CAD build for the part. Positions are in the model's coordinates, mm. Face numbers are marked on the shaded views. A direction names the side the tool comes from. Give positions to 0.01 mm unless a question says otherwise; leave off trailing zeros. Loops run counter-clockwise (first coordinate to the right, second up) from the corner with the lowest first, then second, coordinate; pieces in that order, holes last. Notation, with made-up numbers: (67.25, -10.5) -> (87.25, -10.5) arc R28 ccw to (87.25, 16.5) -> close; hole circle Ø2 at (-21, -11.5). An arc over 180 degrees is marked (long way). Write each question's results on one line, items separated by ' | '. Start each with the question number.
```python
from build123d import *

# Parameters (mm, degrees)
F0_R     = 8.5
F0_R_2   = 5
F1_DEPTH = 6
F2_DEPTH = 11.5
F4_D     = 3.3
F4_DEPTH = 10.001
F5_D     = 3.3


with BuildPart() as f1:
    # F0 (on Front) → F1 (new body)
    with BuildSketch(Plane.XZ):
        with BuildLine():
            Line((-1.5, 11.9058808998), (-5, 8.6602540378))
            ThreePointArc((-5, 8.6602540378), (0, -10), (5, 8.6602540378))
            Line((5, 8.6602540378), (1.5, 11.9058808998))
            ThreePointArc((1.5, 11.9058808998), (0, 12), (-1.5, 11.9058808998))
        make_face()
        Circle(F0_R, mode=Mode.SUBTRACT)
        Circle(F0_R)
        Circle(F0_R_2, mode=Mode.SUBTRACT)
    extrude(amount=F1_DEPTH)

    # F0 (on Front) → F2 (join)
    with BuildSketch(Plane.XZ):
        Circle(F0_R)
        Circle(F0_R_2, mode=Mode.SUBTRACT)
    extrude(amount=F2_DEPTH)

    # F4 (through all, one way)
    with BuildSketch(Plane.YZ):
        with Locations((-8.75, 0)):
            Circle(F4_D / 2)
    extrude(amount=-F4_DEPTH, mode=Mode.SUBTRACT)

    # F5 (through all)
    with Locations(Plane(origin=(0, 0, 0), x_dir=(0, 1, 0), z_dir=(-1, 0, 0))):
        with Locations((-8.75, 0)):
            Hole(F5_D / 2)


solid = f1.part
```
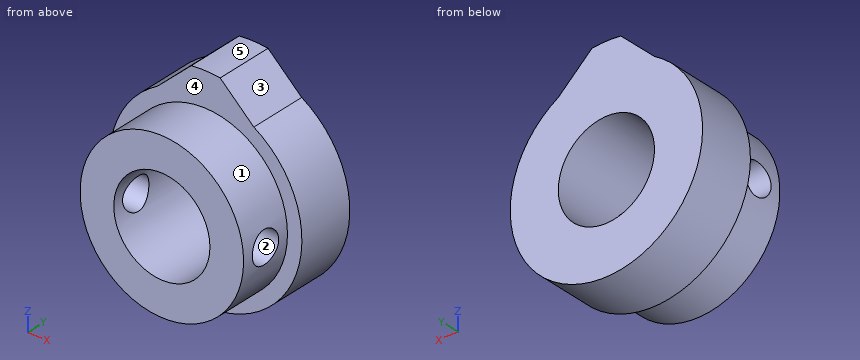
Q1. Mould opens along Z. For the marked faces 1, 2 and 3 say: pulls with the +Z half, pulls with the -Z half, needs draft (parallel to the pull), parting line crosses it, or undercut.
Q2. Saw through at B-B, the plane z = 0.5. List the corners of the cut face in (x, y).
Q3. Saw through at A-A, the plane x = 0. List the corners of the cut face in (y, z), then the cut area to 4 significant figures.
Q4. Saw through at C-C, the plane y = -8.75. List the corners of the cut face in (x, z), then the cut area to 3 significant figures.
Q5. Saw through at D-D, the plane z = -3.75. List the corners of the cut face in (x, y).
Q6. Wall check: L1, parallel to Z at x = 0, y = -3.5; L2, parallel to Z at x = 3.5, y = -6.25; L3, parallel to X at y = -2.25, z = 0. Give the ranges that are in metal, low to high.
Q7. Drop flat-ended pins along their axis: pin 1 (4 mm diameter, centred on x = -5.5, y = -8.5, fed in from -Z); pin 2 (8 mm diameter, centred on x = -3.5, z = 4, fed in from +Y); pin 3 (2 mm diameter, centred on y = -10, z = 4.5, fed in from -X); pin 4 (2 mm diameter, centred on x = -3.5, z = 9, fed in from -Y). Give the stop position or say it passes through.
Q8. Which spindle directions (+Z, -Z, +X, -X, +Y, -Y) get a long thin tool onto all of the face, cutting with end or side? Do the marked faces 4 and 5. Say none if no direction does.
Answer block:
1) face 1: parting line crosses it | face 2: undercut | face 3: pulls with the +Z half
2) outline: (-9.99, -6) -> (-8.49, -6) -> (-8.49, -7.18) -> (-4.97, -7.18) -> (-4.97, 0) -> (-9.99, 0) -> close; (-8.49, -11.5) -> (-4.97, -11.5) -> (-4.97, -10.32) -> (-8.49, -10.32) -> close; (4.97, -11.5) -> (8.49, -11.5) -> (8.49, -10.32) -> (4.97, -10.32) -> close; (4.97, -7.18) -> (8.49, -7.18) -> (8.49, -6) -> (9.99, -6) -> (9.99, 0) -> (4.97, 0) -> close
3) outline: (-11.5, -8.5) -> (-6, -8.5) -> (-6, -10) -> (0, -10) -> (0, -5) -> (-11.5, -5) -> close; (-11.5, 5) -> (0, 5) -> (0, 12) -> (-6, 12) -> (-6, 8.5) -> (-11.5, 8.5) -> close | area: 110.5 mm2
4) outline: (-8.34, -1.65) arc R8.5 ccw to (8.34, -1.65) -> (4.72, -1.65) arc R5 cw to (-4.72, -1.65) -> close; (-8.34, 1.65) -> (-4.72, 1.65) arc R5 cw to (4.72, 1.65) -> (8.34, 1.65) arc R8.5 ccw to start | area: 125 mm2
5) outline: (-9.27, -6) -> (-7.63, -6) -> (-7.63, -11.5) -> (-3.31, -11.5) -> (-3.31, 0) -> (-9.27, 0) -> close; (3.31, -11.5) -> (7.63, -11.5) -> (7.63, -6) -> (9.27, -6) -> (9.27, 0) -> (3.31, 0) -> close
6) L1: z = -10 to -5, 5 to 12 | L2: z = -7.75 to -3.57, 3.57 to 7.75 | L3: x = -10 to -5, 5 to 10
7) pin 1: stops at z = -7.75 | pin 2: stops at y = 0 | pin 3: stops at x = -7.75 | pin 4: stops at y = -6
8) face 4: -Y | face 5: +Z, +Y, -Y
